Source: CAD feature listing. Evaluate the final solid. Frame: model axes, mm. A direction names the side the tool comes from. Coordinates: 2 decimals unless noted, no trailing zeros. Loops run counter-clockwise (first coordinate to the right, second up) from the corner with the lowest first, then second, coordinate; pieces in that order, holes last.
Item 1: Section query A-A, the plane z = 18. Return the cut outline in (x, y) (3 decimals).
Item 2: Pull-direction query (Z, two-part tool) for faces 4 (the cylindrical face through (-0.633, 2.852, 84.704)), 5 (the flat face through (0, 0, 87.569)), 6 (the cylindrical face through (-0.69, -3.1, 86.31)); classes: +Z half, -Z half, draft (parallel to the pull), parting line (faces both ways), or undercut.
Item 3: Line query: probe 1 along Z at (x, y) = (2.5, 1.75); probe 2 along X at (y, z) = (1.25, 16.5); probe 3 along X at (y, z) = (-0.25, 19). Output: solid intervals per line, ascending.
Item 4: Section query B-B, the plane x = 0.75. Return the cut outline in (y, z).
Item 5: Reachability of faces 1 (the flat face through (0, 2.159, 3)), 2 (the cylindrical face through (-0.633, 2.852, 20.363)), 3 (the cylindrical face through (-0.69, -3.1, 52.09)) from +Z, -Z, +X, -X, +Y, -Y: full face, straight path, thin tool, end or side. Return the list, or none.
Item 6: Pin query (flat end, axial travel): pin 1 Ø1.5 at (y, z) = (1, 15) entering from +X; pin 2 Ø0.8 at (x, y) = (-0.5, 3) entering from -Z; pin 3 Ø1.9 at (x, y) = (1, -1.5) entering from -Z; pin 4 Ø1.4 at (x, z) = (0.5, 2.5) entering from +Y. Return the tip coordinate at first contact, or that it passes through.
```python
from build123d import *

# Parameters (mm, degrees)
F0_R     = 3.175
F1_DEPTH = 87.5692
F3_R     = 3.175
F3_R_2   = 2.921
F4_DEPTH = 0.7366
F6_R     = 3.175
F6_R_2   = 2.921
F7_DEPTH = 0.7366
F9_DEPTH = 6.35


# Not quite as in the source:
# - a length typed as a fraction of an inch, garbled in the dataset ("3 / 203.2 mm" for 3/8 in), is restored


with BuildPart() as f1:
    # F0 (on Top) → F1 (new body)
    with BuildSketch(Plane.XY):
        Circle(F0_R)
    extrude(amount=F1_DEPTH)

    # F3 (on offset) → F4 (cut)
    with BuildSketch(Plane(origin=(0, 0, 20), x_dir=(1, 0, 0), z_dir=(0, 0, -1))):
        Circle(F3_R)
        Circle(F3_R_2, mode=Mode.SUBTRACT)
    extrude(amount=-F4_DEPTH, mode=Mode.SUBTRACT)

    # F6 (on offset) → F7 (cut)
    with BuildSketch(Plane(origin=(0, 0, 84.3406), x_dir=(1, 0, 0), z_dir=(0, 0, -1))):
        Circle(F6_R)
        Circle(F6_R_2, mode=Mode.SUBTRACT)
    extrude(amount=-F7_DEPTH, mode=Mode.SUBTRACT)

    # F8 (on face) → F9 (cut)
    with BuildSketch(Plane(origin=(0, 0, 0), x_dir=(1, 0, 0), z_dir=(0, 0, -1))):
        with BuildLine():
            Line((2.327948453, -2.159), (-2.327948453, -2.159))
            ThreePointArc((-2.327948453, -2.159), (0, -3.175), (2.327948453, -2.159))
        make_face()
    extrude(amount=-F9_DEPTH, mode=Mode.SUBTRACT)


solid = f1.part
```
Verdict:
1. outline: circle Ø6.35 at (0, 0)
2. face 4: undercut
2. face 5: +Z half
2. face 6: draft
3. probe 1: z = 0 to 20, 20.74 to 84.34, 85.08 to 87.57
3. probe 2: x = -2.92 to 2.92
3. probe 3: x = -3.17 to 3.17
4. outline: (-3.09, 0) - (2.16, 0) - (2.16, 6.35) - (3.09, 6.35) - (3.09, 20) - (2.82, 20) - (2.82, 20.74) - (3.09, 20.74) - (3.09, 84.34) - (2.82, 84.34) - (2.82, 85.08) - (3.09, 85.08) - (3.09, 87.57) - (-3.09, 87.57) - (-3.09, 85.08) - (-2.82, 85.08) - (-2.82, 84.34) - (-3.09, 84.34) - (-3.09, 20.74) - (-2.82, 20.74) - (-2.82, 20) - (-3.09, 20) - close
5. face 1: -Z, +X, -X, +Y
5. face 2: none
5. face 3: +Z, -Z
6. pin 1: stops at x = 3.17
6. pin 2: stops at z = 6.35
6. pin 3: stops at z = 0
6. pin 4: stops at y = 2.16
